Verification items for the finished model (mm, model axes). Face numbers are marked on the shaded views. Give positions to 0.01 mm unless a question says otherwise; leave off trailing zeros. Loops run counter-clockwise (first coordinate to the right, second up) from the corner with the lowest first, then second, coordinate; pieces in that order, holes last. Notation, with made-up numbers: M -3.5,-33.5 L 5.5,-33.5 A15 cw 5.5,-14.5 Z; hole C -39,58 d7. An arc over 180 degrees is marked long. Put each result on its own line as item: value. Start each with the question number.
from build123d import *

# Parameters (mm, degrees)
F0_W        = 50
F0_H        = 23
F1_DEPTH    = 1.5
F2_W        = 45
F2_H        = 18
F3_DEPTH    = 2
F4_T        = 1.2
F4_T3_DEPTH = 47.4
F4_T5_DEPTH = 20.4


# Not quite as in the source:
# - a shell that OpenCascade refuses in one call is made with other operations: the cavity is built on its own and cut out


with BuildPart() as f1:
    # F0 (on Top) → F1 (new body)
    with BuildSketch(Plane.XY):
        Rectangle(F0_W, F0_H)
    extrude(amount=F1_DEPTH)

    # F2 (on face) → F3 (join)
    with BuildSketch(Plane.XY.offset(1.5)):
        Rectangle(F2_W, F2_H)
    extrude(amount=F3_DEPTH)

    # F4: shell of thickness 1.2, made by hand


with BuildPart() as f4_core1:
    # F4_t2: copy of F1
    add(f1.part)

    # the walls: a layer under each face that stays
    f4_faces = [f4_core1.faces().sort_by_distance(p)[0] for p in [
        (0, 11.5, 0.75),
        (25, 0, 0.75),
        (-25, 0, 0.75),
        (0, 0, 0),
        (-21.4285714286, -9.8571428571, 1.5),
        (0, -11.5, 0.75),
        (0, 9, 2.5),
        (-22.5, 0, 2.5),
        (0, -9, 2.5),
        (22.5, 0, 2.5),
    ]]
    thicken(f4_faces, amount=-F4_T, mode=Mode.SUBTRACT)

    # F4_s4 → F4_t3 (cut)
    with BuildSketch(Plane.YZ.offset(-23.7)):
        Polygon((9.012, 1.512), (9, 0.3), (7.8, 0.3), (7.8, 1.5), align=None)
        Polygon((-9.012, 1.512), (-9, 0.3), (-7.8, 0.3), (-7.8, 1.5), align=None)
    extrude(amount=F4_T3_DEPTH, mode=Mode.SUBTRACT)

    # F4_s6 → F4_t5 (cut)
    with BuildSketch(Plane.XZ.offset(-10.2)):
        Polygon((-22.512, 1.512), (-22.5, 0.3), (-21.3, 0.3), (-21.3, 1.5), align=None)
        Polygon((22.512, 1.512), (22.5, 0.3), (21.3, 0.3), (21.3, 1.5), align=None)
    extrude(amount=F4_T5_DEPTH, mode=Mode.SUBTRACT)


with BuildPart() as f1_1:
    add(f1.part)

    # what is left inside the walls is the cavity
    f4_cavity = [f4_core1.part.solids().sort_by_distance(p)[0] for p in [
        (0, -2.6, 3.488),
    ]]
    add(f4_cavity, mode=Mode.SUBTRACT)


solid = f1_1.part
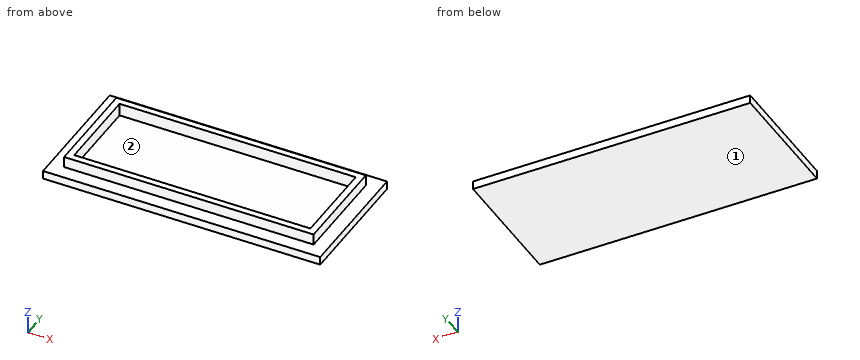
Q1. Cross-section at B-B, the plane z = 2.7. Record the boundary of the cut face in (x, y), then the cut area to 3 significant figures.
Q2. Go/stop test with flat-tipped pins: pin 1 (1.6 mm diameter, centred on x = 6.5, z = 2, fed in from -Y); pin 2 (4.5 mm diameter, centred on x = -6, y = -2, fed in from +Z); pin 3 (1.6 mm diameter, centred on y = -1.5, z = 2.5, fed in from -X); pin 4 (1 mm diameter, centred on x = -4.5, z = 2.5, fed in from +Y). Record where each tip stops, or that it passes through.
Q3. Release check for a two-part mould opening along X. For the marked faces 1 and 2 record: pulls with the +X half, pulls with the -X half, needs draft (parallel to the pull), parting line crosses it, or undercut.
Q4. Cross-section at A-A, the plane x = -8.5. Record the boundary of the cut face in (y, z), then the cut area to 3 significant figures.
Q5. Cross-section at C-C, the plane y = 7. Record the boundary of the cut face in (x, z).
Q6. Scan lines: L1, parallel to X at y = -1.25, z = 3.15; L2, parallel to Y at x = -5.5, z = 1.95; L3, parallel to Z at x = -14, y = -3. Record each from-to range of solid material in increasing order.
Q7. Cross-section at D-D, the plane x = 22. Record the boundary of the cut face in (y, z).
Ans:
1. outline: M -22.5,-9 L 22.5,-9 L 22.5,9 L -22.5,9 Z; hole M -21.3,-7.8 L 21.3,-7.8 L 21.3,7.8 L -21.3,7.8 Z
1. area: 145 mm^2
2. pin 1: stops at y = -11.5
2. pin 2: stops at z = 1.2
2. pin 3: stops at x = -22.5
2. pin 4: stops at y = 9
3. face 1: needs draft
3. face 2: undercut
4. outline: M -11.5,0 L 11.5,0 L 11.5,1.5 L 9,1.5 L 9,3.5 L 7.8,3.5 L 7.8,1.2 L -7.8,1.2 L -7.8,3.5 L -9,3.5 L -9,1.5 L -11.5,1.5 Z
4. area: 34.6 mm^2
5. outline: M -25,0 L 25,0 L 25,1.5 L 22.5,1.5 L 22.5,3.5 L 21.3,3.5 L 21.3,1.2 L -21.3,1.2 L -21.3,3.5 L -22.5,3.5 L -22.5,1.5 L -25,1.5 Z
6. L1: x = -22.5 to -21.3, 21.3 to 22.5
6. L2: y = -9 to -7.8, 7.8 to 9
6. L3: z = 0 to 1.2
7. outline: M -11.5,0 L 11.5,0 L 11.5,1.5 L 9,1.5 L 9,3.5 L -9,3.5 L -9,1.5 L -11.5,1.5 Z
